Read the model definition and answer for the solid it produces. Units are mm, in the model's axes. A direction names the side the tool comes from. Give positions to 0.01 mm unless a question says otherwise; leave off trailing zeros. Order: outer loops, then holes, each group sorted by start corner. A loop starts at its lowest first (then second) coordinate and runs counter-clockwise, first axis right, second up. Notation, with made-up numbers: M 49,8.25 L 103,8.25 A29 cw 103,34.25 Z; hole C 72,-12 d5. An arc over 180 degrees is marked long. One line per item, written item: value.
from build123d import *

# Parameters (mm, degrees)
F0_W      = 37
F0_H      = 24.3
F0_W_2    = 31
F0_H_2    = 9.15
F1_DEPTH  = 3
F2_DEPTH  = 13
F3_W      = 3
F3_H      = 18.3
F4_DEPTH  = 13
F5_W      = 28.5
F5_H      = 13.3
F5_W_2    = 3
F6_DEPTH  = 3
F7_W      = 22
F7_H      = 5
F8_DEPTH  = 12
F10_R     = 5
F11_DEPTH = 25


with BuildPart() as f1:
    # F0 (on Front) → F1 (new body)
    with BuildSketch(Plane.XZ):
        with Locations((15.5, 9.15)):
            Rectangle(F0_W, F0_H)
        Polygon((31, 0), (0, 0), (0, 9.15), (0, 18.3), (31, 18.3), (31, 9.15), align=None, mode=Mode.SUBTRACT)
        with Locations((15.5, 13.725)):
            Rectangle(F0_W_2, F0_H_2)
        with Locations((15.5, 4.575)):
            Rectangle(F0_W_2, F0_H_2)
    extrude(amount=-F1_DEPTH)

    # F0 (on Front) → F2 (join)
    with BuildSketch(Plane.XZ):
        with Locations((15.5, 9.15)):
            Rectangle(F0_W, F0_H)
        Polygon((31, 0), (0, 0), (0, 9.15), (0, 18.3), (31, 18.3), (31, 9.15), align=None, mode=Mode.SUBTRACT)
    extrude(amount=F2_DEPTH)

    # F3 (on face) → F4 (cut, through all)
    with BuildSketch(Plane.XZ.offset(13)):
        with Locations((32.5, 9.15)):
            Rectangle(F3_W, F3_H)
    extrude(amount=-F4_DEPTH, mode=Mode.SUBTRACT)

    # F5 (on face) → F6 (join)
    with BuildSketch(Plane.XZ):
        with Locations((16.75, 9.15)):
            Rectangle(F5_W, F5_H)
        with Locations((32.5, 9.15)):
            Rectangle(F5_W_2, F5_H)
    extrude(amount=F6_DEPTH)

    # F7 (on face) → F8 (join)
    with BuildSketch(Plane(origin=(0, 0, -3), x_dir=(1, 0, 0), z_dir=(0, 0, -1))):
        with Locations((15.5, -0.5)):
            Rectangle(F7_W, F7_H)
    extrude(amount=F8_DEPTH)

    # F10
    f10_edges = [f1.edges().sort_by_distance(p)[0] for p in [
        (4.5, 0.5, -15),
        (4.5, 0.5, -3),
        (26.5, 0.5, -15),
        (26.5, 0.5, -3),
    ]]
    fillet(f10_edges, radius=F10_R)

    # F9 (on face) → F11 (cut)
    with BuildSketch(Plane.XZ.offset(2)):
        with BuildLine():
            Line((8.5, -9), (12.5, -9))
            ThreePointArc((12.5, -9), (10.5, -7), (8.5, -9))
        make_face()
        with BuildLine():
            ThreePointArc((8.5, -9), (10.5, -11), (12.5, -9))
            Line((12.5, -9), (8.5, -9))
        make_face()
        with BuildLine():
            Line((18.5, -9), (22.5, -9))
            ThreePointArc((22.5, -9), (20.5, -7), (18.5, -9))
        make_face()
        with BuildLine():
            ThreePointArc((18.5, -9), (20.5, -11), (22.5, -9))
            Line((22.5, -9), (18.5, -9))
        make_face()
    extrude(amount=-F11_DEPTH, mode=Mode.SUBTRACT)


solid = f1.part
1) Consider probe 1 along X at (y, z) = (1.15, -9); probe 2 along Z at (x, y) = (17, -2.5); probe 3 along Z at (x, y) = (1, -2.5). Determine where each line is inside the solid, lowest interval first.
Reported:
probe 1: x = 4.5 to 8.5, 12.5 to 18.5, 22.5 to 26.5
probe 2: z = -3 to 0, 2.5 to 15.8, 18.3 to 21.3
probe 3: z = -3 to 0, 18.3 to 21.3
2) Find section C-C, the plane x = 20.5. Write down the section's boundary in (y, z).
Reported:
outline: M -13,-3 L -2,-3 L -2,-7 L 3,-7 L 3,21.3 L -13,21.3 L -13,18.3 L 0,18.3 L 0,15.8 L -3,15.8 L -3,2.5 L 0,2.5 L 0,0 L -13,0 Z; M -2,-15 L 3,-15 L 3,-11 L -2,-11 Z
3) Each of these flat-tipped pins is pushed along its axis until it touches: pin 1 Ø6 at (x, z) = (7.5, -11) entering from -Y; pin 2 Ø0.6 at (y, z) = (1, -9.5) entering from +X; pin 3 Ø9 at (x, z) = (13.5, 13) entering from -Y; pin 4 Ø3.5 at (x, z) = (10.5, -9) entering from -Y. Where does it stop, or does it pass through?
Reported:
pin 1: stops at y = -2
pin 2: stops at x = 26.5
pin 3: stops at y = -3
pin 4: passes through
4) Find section A-A, the plane y = -1.5. Write down the section's boundary in (x, z), plus the area to 3 significant figures.
Reported:
outline: M -3,-3 L -0.5,-3 A5 cw 4.5,-8 L 4.5,-10 A5 ccw 9.5,-15 L 21.5,-15 A5 ccw 26.5,-10 L 26.5,-8 A5 cw 31.5,-3 L 34,-3 L 34,0 L 0,0 L 0,18.3 L 34,18.3 L 34,21.3 L -3,21.3 Z; M 2.5,2.5 L 34,2.5 L 34,15.8 L 2.5,15.8 Z; hole C 10.5,-9 d4; hole C 20.5,-9 d4
area: 935 mm^2
5) Find section D-D, the plane x = 5.5. Write down the section's boundary in (y, z).
Reported:
outline: M -13,-3 L -2,-3 L -2,-13 L 3,-13 L 3,21.3 L -13,21.3 L -13,18.3 L 0,18.3 L 0,15.8 L -3,15.8 L -3,2.5 L 0,2.5 L 0,0 L -13,0 Z
6) Find section B-B, the plane z = -9. Write down the section's boundary in (x, y), plus the area to 3 significant figures.
Reported:
outline: M 4.5,-2 L 8.5,-2 L 8.5,3 L 4.5,3 Z; M 12.5,-2 L 18.5,-2 L 18.5,3 L 12.5,3 Z; M 22.5,-2 L 26.5,-2 L 26.5,3 L 22.5,3 Z
area: 70.0 mm^2
7) Determine the mould class of faces 4 (the face through (34, -1, 9)), 5 (the face through (2.5, -1, 9)), 6 (the face through (15, -7, -3)) for opening direction X: +X half, -X half, draft (parallel to the pull), parting line (faces both ways), or undercut.
Reported:
face 4: +X half
face 5: undercut
face 6: draft
8) Which of the six approach directions +Z, -Z, +X, -X, +Y, -Y give full straight-line access (tool end or side, diameter ignored) to faces 1 (the face through (4.5, 1, -9)), 2 (the face through (26.5, 1, -9)), 3 (the face through (18, -1, 2.5))?
Reported:
face 1: -Z, -X, +Y, -Y
face 2: -Z, +X, +Y, -Y
face 3: +X, -Y
